```python
from build123d import *

# Parameters (mm, degrees)
F1_DEPTH = 20
F2_W     = 25
F2_H     = 15
F3_DEPTH = 20
F4_R     = 2.5
F5_DEPTH = 20


with BuildPart() as f1:
    # F0 (on Right) → F1 (new body)
    with BuildSketch(Plane.YZ):
        with BuildLine():
            ThreePointArc((122.5, -17.5), (140, 0), (122.5, 17.5))
            Line((122.5, 17.5), (-140, 17.5))
            Line((-140, 17.5), (-115, -17.5))
            Line((-115, -17.5), (122.5, -17.5))
        make_face()
    extrude(amount=F1_DEPTH)

    # F2 (on face) → F3 (cut)
    with BuildSketch(Plane.YZ.offset(20)):
        with Locations((-52.5, 10)):
            Rectangle(F2_W, F2_H)
        with Locations((67.5, 10)):
            Rectangle(F2_W, F2_H)
    extrude(amount=-F3_DEPTH, mode=Mode.SUBTRACT)

    # F4 (on face) → F5 (cut)
    with BuildSketch(Plane.YZ.offset(20)):
        with Locations((122.5, 0)):
            Circle(F4_R)
    extrude(amount=-F5_DEPTH, mode=Mode.SUBTRACT)


solid = f1.part
```
Here's how the part is built. I have some questions about the finished solid (model axes, mm). A direction names the side the tool comes from. Coordinates: 2 decimals unless noted, no trailing zeros. Write each loop counter-clockwise with the first axis right and the second up, starting at its lowest first coordinate (ties: lowest second). Pieces come first, ordered by that corner, then holes. Notation, with made-up numbers: (-35, 21.25) -> (-1, 21.25) arc R33 ccw to (-1, 49.25) -> close; hole circle Ø4 at (-9, 30.25). An arc over 180 degrees is marked (long way). Use a Markdown table: item, result. Add a question column.
(1) If we section it at C-C, the plane z = 13: Write out the boundary of the cut face in (x, y).
(2) If we section it at B-B, the plane x = 14: Write out the boundary of the cut face in (y, z).
(3) For faces 1 (the flat face through (10, 80, 10)), 2 (the flat face through (10, 102, 17.5)), which set-ups out of +Z, -Z, +X, -X, +Y, -Y let a thin tool reach every point of the face, with its end or its side?
(4) If we section it at A-A, the plane z = 0: Write out the boundary of the cut face in (x, y).
(5) Please list where these lines run through material, in increasing order: line 1 (Z direction, x = 6.75, y = 122.5); line 2 (Y direction, x = 2, z = 3.5); line 3 (Y direction, x = 7.25, z = 3).
(6) If we section it at D-D, the plane y = -59: Write out the boundary of the cut face in (x, z), and give its area (3 significant figures).
(7) We'd pull the mould along Y, two halves only. Please class faces 3 (the cylindrical face through (10, 140, 0)), 4 (the flat face through (10, 8, 17.5)), 5 (the flat face through (10, 67, 2.5)), 6 (the flat face through (10, -40, 10)): +Y half, -Y half, draft (parallel to the pull), parting line (faces both ways), or undercut.
(8) I'm going to push flat-ended pins straight in: P1, Ø1, axis at x = 12.5, z = 10.5, coming from the -Y side; P2, Ø4.5, axis at x = 11.5, z = 12.5, coming from the +Y side; P3, Ø12, axis at x = 14.5, z = 0.5, coming from the -Y side. Where does each tip first touch, or does it pass through?
Outcome:
| question | item | result |
|---|---|---|
| 1 | outline | (0, -136.79) -> (20, -136.79) -> (20, -65) -> (0, -65) -> close; (0, -40) -> (20, -40) -> (20, 55) -> (0, 55) -> close; (0, 80) -> (20, 80) -> (20, 134.22) -> (0, 134.22) -> close |
| 2 | outline | (-140, 17.5) -> (-115, -17.5) -> (122.5, -17.5) arc R17.5 ccw to (122.5, 17.5) -> (80, 17.5) -> (80, 2.5) -> (55, 2.5) -> (55, 17.5) -> (-40, 17.5) -> (-40, 2.5) -> (-65, 2.5) -> (-65, 17.5) -> close; hole circle Ø5 at (122.5, 0) |
| 3 | face 1 | +Z, +X, -X |
| 3 | face 2 | +Z, +X, -X, +Y, -Y |
| 4 | outline | (0, -127.5) -> (20, -127.5) -> (20, 120) -> (0, 120) -> close; (0, 125) -> (20, 125) -> (20, 140) -> (0, 140) -> close |
| 5 | line 1 | z = -17.5 to -2.5, 2.5 to 17.5 |
| 5 | line 2 | y = -130 to -65, -40 to 55, 80 to 139.65 |
| 5 | line 3 | y = -129.64 to -65, -40 to 55, 80 to 139.74 |
| 6 | outline | (0, -17.5) -> (20, -17.5) -> (20, 2.5) -> (0, 2.5) -> close |
| 6 | area | 400 mm^2 |
| 7 | face 3 | +Y half |
| 7 | face 4 | draft |
| 7 | face 5 | undercut |
| 7 | face 6 | undercut |
| 8 | P1 | stops at y = -135.36 |
| 8 | P2 | stops at y = 136.68 |
| 8 | P3 | stops at y = -132.14 |
